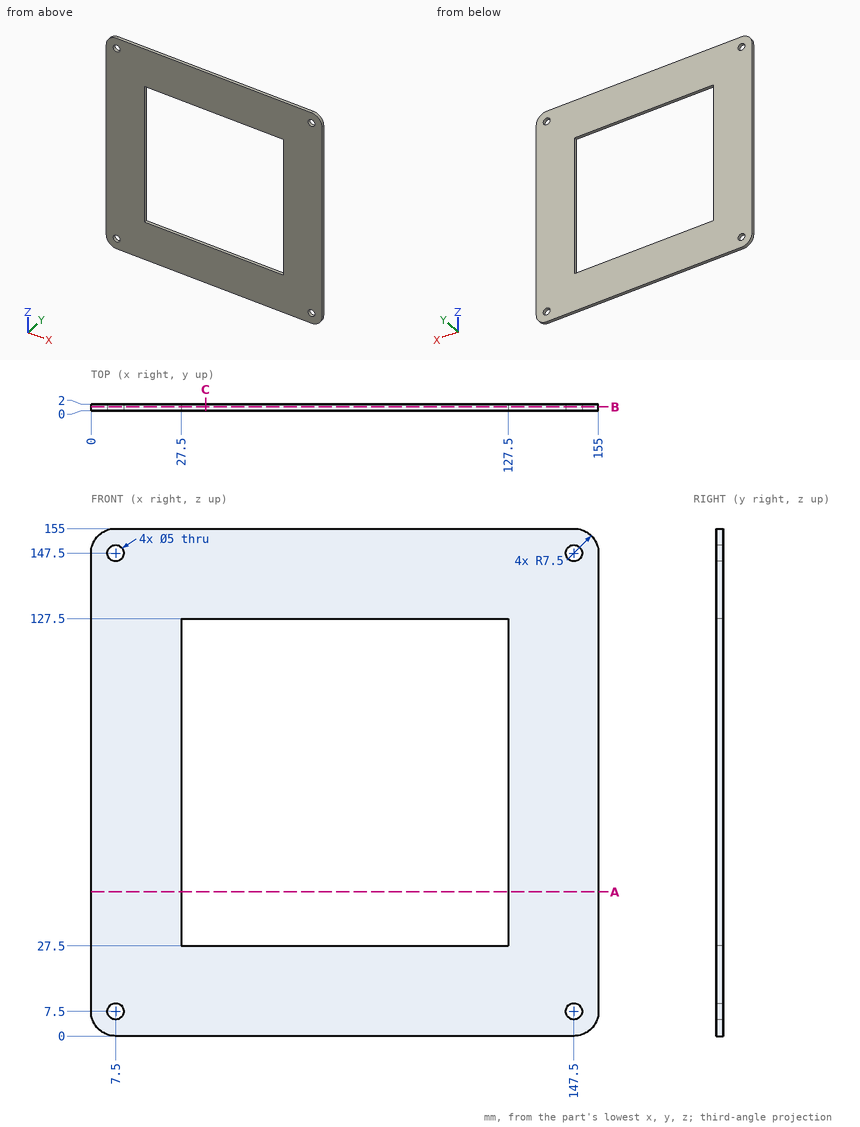
Geometry: see drawing. Coordinates: mm, zero at the bounding-box minimum. Coordinates: 2 decimals unless noted, no trailing zeros. Order: outer loops, then holes, each group sorted by start corner. A loop starts at its lowest first (then second) coordinate and runs counter-clockwise, first axis right, second up. Notation, with made-up numbers: (3.25, -11) - (49.25, -11) arc R21 ccw to (49.25, 11) - close; hole circle Ø4 at (32, 64.25). An arc over 180 degrees is marked (long way). Write each question's results on one line, items separated by ' | '.
1) Line query: line 1 (X direction, y = 0.45, z = 147.5); line 2 (X direction, y = 1.1, z = 30.5). Output: solid intervals per line, ascending. Write a range as from..to.
Results list:
line 1: 0..5, 10..145, 150..155 | line 2: 0..27.5, 127.5..155
2) Section A-A, the plane z = 44. Return loops of the section in (x, y), plus the area to 3 significant figures.
Results list:
outline: (0, 0) - (27.5, 0) - (27.5, 2) - (0, 2) - close; (127.5, 0) - (155, 0) - (155, 2) - (127.5, 2) - close | area: 110 mm^2
3) Section B-B, the plane y = 1.1. Return loops of the section in (x, z), plus the area to 3 significant figures.
Results list:
outline: (0, 7.5) arc R7.5 ccw to (7.5, 0) - (147.5, 0) arc R7.5 ccw to (155, 7.5) - (155, 147.5) arc R7.5 ccw to (147.5, 155) - (7.5, 155) arc R7.5 ccw to (0, 147.5) - close; hole circle Ø5 at (7.5, 7.5); hole circle Ø5 at (7.5, 147.5); hole (27.5, 27.5) - (127.5, 27.5) - (127.5, 127.5) - (27.5, 127.5) - close; hole circle Ø5 at (147.5, 7.5); hole circle Ø5 at (147.5, 147.5) | area: 13,900 mm^2
4) Section C-C, the plane x = 35. Return loops of the section in (y, z).
Results list:
outline: (0, 0) - (2, 0) - (2, 27.5) - (0, 27.5) - close; (0, 127.5) - (2, 127.5) - (2, 155) - (0, 155) - close
